Check sheet for the modelled part. Datum: model origin and axes. Units: mm. A direction names the side the tool comes from. Coordinates: 2 decimals unless noted, no trailing zeros. Order: outer loops, then holes, each group sorted by start corner. A loop starts at its lowest first (then second) coordinate and runs counter-clockwise, first axis right, second up.
1. Thickness scan on line 1 (Y direction, x = 1, z = 0); line 2 (Y direction, x = -14.5, z = 7.5); line 3 (Z direction, x = 0, y = -18.25). Record the ranges inside material, lowest first.
2. Cross-section at B-B (z = -15.5). Enter the section's corners in (x, y), then the cut area to 3 significant figures.
3. Draft check along X on faces 4 (the flat face through (0, -25, 1)), 5 (the cylindrical face through (2.14, -4.93, 2.1)), 6 (the cylindrical face through (10.382, -4.93, -19.961)). Enter one of: released by +X, released by -X, zero draft, split by the parting line, or undercut.
4. Cross-section at C-C (x = -8.5). Enter the section's corners in (y, z).
5. Gauge pin test, flat ends, axial feed: pin 1 Ø1.4 at (x, z) = (0, 0) entering from -Y; pin 2 Ø3 at (y, z) = (-3.5, -2) entering from +X; pin 3 Ø5 at (x, y) = (9, -6) entering from -Z; pin 4 Ø5 at (x, z) = (9, -5.5) entering from +Y. Record the tip position at first contact, or that the pin passes through.
6. Set-up check for faces 1 (the flat face through (0, -15, 0)), 2 (the flat face through (0, 0, 0)), 3 (the flat face through (0, -5, -11)): record each of +Z, -Z, +X, -X, +Y, -Y from which the full face is reachable in a straight line by a thin tool's end or side.
7. Cross-section at A-A (y = -16.5). Enter the section's corners in (x, z).
```python
from build123d import *

# Parameters (mm, degrees)
F0_R     = 22.5
F1_DEPTH = 10
F2_DEPTH = 25
F4_R     = 0.5
F5_DEPTH = 2.5
F6_R     = 0.75
F7_DEPTH = 10


with BuildPart() as f1:
    # F0 (on Front) → F1 (new body)
    with BuildSketch(Plane.XZ):
        Circle(F0_R)
        with BuildLine():
            ThreePointArc((0, 20), (14.1421356237, 14.1421356237), (20, 0))
            ThreePointArc((20, 0), (14.1421356237, -14.1421356237), (0, -20))
            ThreePointArc((0, -20), (-14.1421356237, -14.1421356237), (-20, 0))
            ThreePointArc((-20, 0), (-14.1421356237, 14.1421356237), (0, 20))
        make_face(mode=Mode.SUBTRACT)
        with BuildLine():
            Line((0, 3), (0, 20))
            ThreePointArc((0, 20), (-14.1421356237, 14.1421356237), (-20, 0))
            Line((-20, 0), (-3, 0))
            ThreePointArc((-3, 0), (-2.1213203436, 2.1213203436), (0, 3))
        make_face()
        with BuildLine():
            Line((0, 1.5), (0, 3))
            ThreePointArc((0, 3), (-2.1213203436, 2.1213203436), (-3, 0))
            Line((-3, 0), (-1.5, 0))
            ThreePointArc((-1.5, 0), (-1.0606601718, 1.0606601718), (0, 1.5))
        make_face()
        with BuildLine():
            Line((1.5, 0), (3, 0))
            ThreePointArc((3, 0), (2.1213203436, 2.1213203436), (0, 3))
            Line((0, 3), (0, 1.5))
            ThreePointArc((0, 1.5), (1.0606601718, 1.0606601718), (1.5, 0))
        make_face()
        with BuildLine():
            ThreePointArc((-3, 0), (-2.1213203436, -2.1213203436), (0, -3))
            Line((0, -3), (0, -1.5))
            ThreePointArc((0, -1.5), (-1.0606601718, -1.0606601718), (-1.5, 0))
            Line((-1.5, 0), (-3, 0))
        make_face()
        with BuildLine():
            ThreePointArc((0, -3), (2.1213203436, -2.1213203436), (3, 0))
            Line((3, 0), (1.5, 0))
            ThreePointArc((1.5, 0), (1.0606601718, -1.0606601718), (0, -1.5))
            Line((0, -1.5), (0, -3))
        make_face()
        with BuildLine():
            ThreePointArc((0, -20), (14.1421356237, -14.1421356237), (20, 0))
            Line((20, 0), (3, 0))
            ThreePointArc((3, 0), (2.1213203436, -2.1213203436), (0, -3))
            Line((0, -3), (0, -20))
        make_face()
    extrude(amount=F1_DEPTH)

    # F0 (on Front) → F2 (join)
    with BuildSketch(Plane.XZ):
        with BuildLine():
            Line((0, 0), (0, 1.5))
            ThreePointArc((0, 1.5), (-1.0606601718, 1.0606601718), (-1.5, 0))
            Line((-1.5, 0), (0, 0))
        make_face()
        with BuildLine():
            ThreePointArc((-1.5, 0), (-1.0606601718, -1.0606601718), (0, -1.5))
            Line((0, -1.5), (0, 0))
            Line((0, 0), (-1.5, 0))
        make_face()
        with BuildLine():
            ThreePointArc((0, -1.5), (1.0606601718, -1.0606601718), (1.5, 0))
            Line((1.5, 0), (0, 0))
            Line((0, 0), (0, -1.5))
        make_face()
        with BuildLine():
            Line((0, 0), (1.5, 0))
            ThreePointArc((1.5, 0), (1.0606601718, 1.0606601718), (0, 1.5))
            Line((0, 1.5), (0, 0))
        make_face()
    extrude(amount=F2_DEPTH)

    # F4 (on face) → F5 (cut)
    with BuildSketch(Plane.YZ):
        with Locations((-23.5, 0)):
            Circle(F4_R)
    extrude(amount=F5_DEPTH, mode=Mode.SUBTRACT)

    # F6 (on face) → F7 (cut)
    with BuildSketch(Plane.XZ.offset(25)):
        Circle(F6_R)
    extrude(amount=-F7_DEPTH, mode=Mode.SUBTRACT)


solid = f1.part
```
Data:
1. line 1: y = -25 to -24, -23 to 0
1. line 2: y = -10 to 0
1. line 3: z = -1.5 to -0.75, 0.75 to 1.5
2. outline: (-16.31, -10) - (-12.64, -10) - (-12.64, 0) - (-16.31, 0) - close; (0, -10) - (16.31, -10) - (16.31, 0) - (0, 0) - close
2. area: 200 mm2
3. face 4: zero draft
3. face 5: undercut
3. face 6: split by the parting line
4. outline: (-10, -20.83) - (0, -20.83) - (0, -18.1) - (-10, -18.1) - close; (-10, 0) - (0, 0) - (0, 20.83) - (-10, 20.83) - close
5. pin 1: stops at y = -15
5. pin 2: stops at x = 22.49
5. pin 3: stops at z = -21.54
5. pin 4: stops at y = 0
6. face 1: -Y
6. face 2: +Z, -Z, +X, -X, +Y
6. face 3: +Y, -Y
7. outline: circle Ø3 at (0, 0); hole circle Ø1.5 at (0, 0)
